The model under review builds one solid part; all positions refer to its coordinate system, in mm. A direction names the side the tool comes from. Coordinates: 2 decimals unless noted, no trailing zeros. Loops run counter-clockwise (first coordinate to the right, second up) from the corner with the lowest first, then second, coordinate; pieces in that order, holes last. Notation, with made-up numbers: M 34,16 L 45,16 A14 ccw 45,31 Z; hole C 20.25,79 d5. An arc over 180 degrees is marked long. One line per item, written item: value.
```python
from build123d import *

# Parameters (mm, degrees)
BOSS_EXTRUDE1_DEPTH = 33.6042
CUT_EXTRUDE1_DEPTH  = 1.397
CHAMFER1_SIZE       = 0.762
SKETCH3_W           = 18.6436
SKETCH3_H           = 2.4892
BOSS_EXTRUDE2_DEPTH = 6.604
SKETCH4_W           = 18.6436
SKETCH4_H           = 2.4892
BOSS_EXTRUDE3_DEPTH = 6.604
FILLET1_R           = 1.27
CUT_EXTRUDE2_DEPTH  = 3.048
SKETCH6_W           = 6.604
SKETCH6_H           = 1.2192
BOSS_EXTRUDE4_DEPTH = 1.905
CUT_EXTRUDE3_DEPTH  = 1.905
BOSS_EXTRUDE5_DEPTH = 3.0988
SKETCH9_R           = 6.731
BOSS_EXTRUDE6_DEPTH = 2.159
SKETCH10_R          = 4.9911
BOSS_EXTRUDE7_DEPTH = 0.508
SKETCH11_R          = 2.8702
BOSS_EXTRUDE8_DEPTH = 3.6576
SKETCH12_R          = 1.0668
CUT_EXTRUDE4_DEPTH  = 5.08
CHAMFER2_SIZE       = 0.254
SCALE1_SCALE        = 0.6


with BuildPart() as part:
    # Sketch1 → Boss-Extrude1 (new body)
    with BuildSketch(Plane(origin=(0, 0, 0), x_dir=(1, 0, 0), z_dir=(0, 1, 0))):
        with BuildLine():
            Line((0, 9.0424), (0, -9.0424))
            ThreePointArc((0, -9.0424), (0.29757951, -9.76082049), (1.016, -10.0584))
            Line((1.016, -10.0584), (39.116, -10.0584))
            ThreePointArc((39.116, -10.0584), (39.83442049, -9.76082049), (40.132, -9.0424))
            Line((40.132, -9.0424), (40.132, 9.0424))
            ThreePointArc((40.132, 9.0424), (39.83442049, 9.76082049), (39.116, 10.0584))
            Line((39.116, 10.0584), (1.016, 10.0584))
            ThreePointArc((1.016, 10.0584), (0.29757951, 9.76082049), (0, 9.0424))
        make_face()
    extrude(amount=BOSS_EXTRUDE1_DEPTH)

    # Sketch2 → Cut-Extrude1 (cut)
    with BuildSketch(Plane.XZ):
        with BuildLine():
            Line((4.6482, 10.0584), (4.6482, 7.3533))
            ThreePointArc((4.6482, 7.3533), (4.067919955, 5.952380045), (2.667, 5.3721))
            Line((2.667, 5.3721), (0, 5.3721))
            Line((0, 5.3721), (0, 9.0424))
            ThreePointArc((0, 9.0424), (0.29757951, 9.76082049), (1.016, 10.0584))
            Line((1.016, 10.0584), (4.6482, 10.0584))
        make_face()
        with BuildLine():
            Line((35.4838, 10.0584), (35.4838, 7.3533))
            ThreePointArc((35.4838, 7.3533), (36.064080045, 5.952380045), (37.465, 5.3721))
            Line((37.465, 5.3721), (40.132, 5.3721))
            Line((40.132, 5.3721), (40.132, 9.0424))
            ThreePointArc((40.132, 9.0424), (39.83442049, 9.76082049), (39.116, 10.0584))
            Line((39.116, 10.0584), (35.4838, 10.0584))
        make_face()
        with BuildLine():
            Line((0, -5.3721), (2.667, -5.3721))
            ThreePointArc((2.667, -5.3721), (4.067919955, -5.952380045), (4.6482, -7.3533))
            Line((4.6482, -7.3533), (4.6482, -10.0584))
            Line((4.6482, -10.0584), (1.016, -10.0584))
            ThreePointArc((1.016, -10.0584), (0.29757951, -9.76082049), (0, -9.0424))
            Line((0, -9.0424), (0, -5.3721))
        make_face()
        with BuildLine():
            Line((37.465, -5.3721), (40.132, -5.3721))
            Line((40.132, -5.3721), (40.132, -9.0424))
            ThreePointArc((40.132, -9.0424), (39.83442049, -9.76082049), (39.116, -10.0584))
            Line((39.116, -10.0584), (35.4838, -10.0584))
            Line((35.4838, -10.0584), (35.4838, -7.3533))
            ThreePointArc((35.4838, -7.3533), (36.064080045, -5.952380045), (37.465, -5.3721))
        make_face()
    extrude(amount=-CUT_EXTRUDE1_DEPTH, mode=Mode.SUBTRACT)

    # Chamfer1
    chamfer1_edges = [part.edges().sort_by_distance(p)[0] for p in [
        (20.066, 0, 10.0584),
        (0, 0, 0),
        (40.132, 0, 0),
        (20.066, 0, -10.0584),
    ]]
    chamfer(chamfer1_edges, length=CHAMFER1_SIZE)

    # Sketch3 → Boss-Extrude2 (add, symmetric)
    with BuildSketch(Plane(origin=(40.132, 0, 0), x_dir=(0, 0, -1), z_dir=(1, 0, 0))):
        with Locations((0, 27.4574)):
            Rectangle(SKETCH3_W, SKETCH3_H)
    extrude(amount=BOSS_EXTRUDE2_DEPTH, both=True)

    # Sketch4 → Boss-Extrude3 (add, symmetric)
    with BuildSketch(Plane.ZY):
        with Locations((0, 27.4574)):
            Rectangle(SKETCH4_W, SKETCH4_H)
    extrude(amount=BOSS_EXTRUDE3_DEPTH, both=True)

    # Fillet1
    fillet1_edges = [part.edges().sort_by_distance(p)[0] for p in [
        (46.736, 27.4574, 9.3218),
        (46.736, 27.4574, -9.3218),
        (-6.604, 27.4574, -9.3218),
        (-6.604, 27.4574, 9.3218),
    ]]
    fillet(fillet1_edges, radius=FILLET1_R)

    # Sketch5 → Cut-Extrude2 (cut)
    with BuildSketch(Plane(origin=(0, 28.702, 0), x_dir=(1, 0, 0), z_dir=(0, 1, 0))):
        with BuildLine():
            Line((-6.604, 3.4925), (-5.625185736, 3.4925))
            ThreePointArc((-5.625185736, 3.4925), (-1.7018, 4.9911), (-5.625185736, 6.4897))
            Line((-5.625185736, 6.4897), (-6.604, 6.4897))
            Line((-6.604, 6.4897), (-6.604, 3.4925))
        make_face()
        with BuildLine():
            Line((-6.604, -6.4897), (-5.625185736, -6.4897))
            ThreePointArc((-5.625185736, -6.4897), (-1.7018, -4.9911), (-5.625185736, -3.4925))
            Line((-5.625185736, -3.4925), (-6.604, -3.4925))
            Line((-6.604, -3.4925), (-6.604, -6.4897))
        make_face()
        with BuildLine():
            Line((45.757185736, -6.4897), (46.736, -6.4897))
            Line((46.736, -6.4897), (46.736, -3.4925))
            Line((46.736, -3.4925), (45.757185736, -3.4925))
            ThreePointArc((45.757185736, -3.4925), (41.8338, -4.9911), (45.757185736, -6.4897))
        make_face()
        with BuildLine():
            Line((45.757185736, 3.4925), (46.736, 3.4925))
            Line((46.736, 3.4925), (46.736, 6.4897))
            Line((46.736, 6.4897), (45.757185736, 6.4897))
            ThreePointArc((45.757185736, 6.4897), (41.8338, 4.9911), (45.757185736, 3.4925))
        make_face()
    extrude(amount=-CUT_EXTRUDE2_DEPTH, mode=Mode.SUBTRACT)

    # Sketch6 → Boss-Extrude4 (add)
    with BuildSketch(Plane(origin=(0, 28.702, 0), x_dir=(1, 0, 0), z_dir=(0, 1, 0))):
        with Locations((-3.302, 0)):
            Rectangle(SKETCH6_W, SKETCH6_H)
        with Locations((43.434, 0)):
            Rectangle(SKETCH6_W, SKETCH6_H)
    extrude(amount=BOSS_EXTRUDE4_DEPTH)

    # Sketch7 → Cut-Extrude3 (cut)
    with BuildSketch(Plane.XY.offset(0.6096)):
        Polygon((40.132, 30.607), (46.736, 28.702), (46.736, 30.607), align=None)
        Polygon((0, 30.607), (-6.604, 28.702), (-6.604, 30.607), align=None)
    extrude(amount=-CUT_EXTRUDE3_DEPTH, mode=Mode.SUBTRACT)

    # Sketch8 → Boss-Extrude5 (add)
    with BuildSketch(Plane(origin=(0, 33.6042, 0), x_dir=(1, 0, 0), z_dir=(0, 1, 0))):
        with BuildLine():
            Line((14.8583952, -8.8392), (34.1122, -8.8392))
            ThreePointArc((34.1122, -8.8392), (34.291805122, -8.764805122), (34.3662, -8.5852))
            Line((34.3662, -8.5852), (34.3662, -3.741254719))
            ThreePointArc((34.3662, -3.741254719), (36.053651663, 0), (34.3662, 3.741254719))
            Line((34.3662, 3.741254719), (34.3662, 8.5852))
            ThreePointArc((34.3662, 8.5852), (34.291805122, 8.764805122), (34.1122, 8.8392))
            Line((34.1122, 8.8392), (14.8583952, 8.8392))
            ThreePointArc((14.8583952, 8.8392), (0, 0), (14.8583952, -8.8392))
        make_face()
    extrude(amount=BOSS_EXTRUDE5_DEPTH)

    # Sketch9 → Boss-Extrude6 (add)
    with BuildSketch(Plane(origin=(0, 36.703, 0), x_dir=(1, 0, 0), z_dir=(0, 1, 0))):
        with Locations(Location((10.0584, 0, 0), (0, 0, 270))):
            Circle(SKETCH9_R)
    extrude(amount=BOSS_EXTRUDE6_DEPTH)

    # Sketch10 → Boss-Extrude7 (add)
    with BuildSketch(Plane(origin=(0, 38.862, 0), x_dir=(1, 0, 0), z_dir=(0, 1, 0))):
        with Locations(Location((10.0584, 0, 0), (0, 0, 270))):
            Circle(SKETCH10_R)
    extrude(amount=BOSS_EXTRUDE7_DEPTH)

    # Sketch11 → Boss-Extrude8 (add)
    with BuildSketch(Plane(origin=(0, 39.37, 0), x_dir=(1, 0, 0), z_dir=(0, 1, 0))):
        with Locations(Location((10.0584, 0, 0), (0, 0, 270))):
            Circle(SKETCH11_R)
    extrude(amount=BOSS_EXTRUDE8_DEPTH)

    # Sketch12 → Cut-Extrude4 (cut)
    with BuildSketch(Plane(origin=(0, 43.0276, 0), x_dir=(1, 0, 0), z_dir=(0, 1, 0))):
        with Locations(Location((10.0584, 0, 0), (0, 0, 270))):
            Circle(SKETCH12_R)
    extrude(amount=-CUT_EXTRUDE4_DEPTH, mode=Mode.SUBTRACT)

    # Chamfer2
    chamfer2_edges = [part.edges().sort_by_distance(p)[0] for p in [
        (10.0584, 43.0276, -2.8702),
        (10.0584, 43.0276, -1.0668),
    ]]
    chamfer(chamfer2_edges, length=CHAMFER2_SIZE)


with BuildPart() as part_1:
    # Scale1: scaled about (19.790017038, 18.508512474, 0)
    add(part.part.scale(SCALE1_SCALE).moved(Location((7.916006815, 7.40340499, 0))))


solid = part_1.part
```
(1) Draft analysis for pull direction X (two halves, no side actions). For faces 1 (the face through (20, 7.403, 0)), 2 (the face through (33.017, 23.888, 2.949)), 3 (the face through (35.958, 23.9, -4.4)), state which applies: pulls with the +X half, pulls with the -X half, needs draft (parallel to the pull), parting line crosses it, or undercut.
Checks:
face 1: needs draft
face 2: undercut
face 3: pulls with the +X half
(2) To check wall thickness, follow L1, parallel to X at y = 31.4, z = 0; L2, parallel to X at y = 26.75, z = 0.25; L3, parallel to Y at x = 20.5, z = -3.5. State the ranges of each line that lie inside material, in increasing order. Write a range as [from, to].
Checks:
L1: [12.23, 13.31], [14.59, 15.67]
L2: [7.92, 32]
L3: [7.4, 29.43]
(3) Add section C-C on x = 34. State the section outline as (y, z) points.
Checks:
outline: M 23.13,-5.59 L 24.62,-5.59 L 24.62,-4.29 L 23.13,-4.29 Z; M 23.13,-1.7 L 24.62,-1.7 L 24.62,-0.37 L 25.19,-0.37 L 25.19,0.37 L 24.62,0.37 L 24.62,1.7 L 23.13,1.7 Z; M 23.13,4.29 L 24.62,4.29 L 24.62,5.59 L 23.13,5.59 Z
(4) Add section A-A on y = 28.5. State the section outline as (x, z) points, then the cut area to 3 significant figures.
Checks:
outline: M 16.83,-5.3 L 28.38,-5.3 A0.15 ccw 28.54,-5.15 L 28.54,-2.24 A2.99 ccw 28.54,2.24 L 28.54,5.15 A0.15 ccw 28.38,5.3 L 16.83,5.3 A6.04 ccw long Z
area: 218 mm^2
(5) Tool access review of faces 4 (the face through (33, 24.625, 2)), 5 (the face through (10.366, 7.817, 3.581)), 6 (the face through (31, 8.242, 5)): name each direction out of +Z, -Z, +X, -X, +Y, -Y from which nothing blocks a thin tool from reaching the whole face with its end or side.
Checks:
face 4: +Z, +X, +Y
face 5: +Z, -X, -Y
face 6: +Z, +X, -Y
(6) Add section D-D on y = 12.25. State the section outline as (x, z) points, then the cut area to 3 significant figures.
Checks:
outline: M 7.92,-5.43 A0.61 ccw 8.53,-6.04 L 31.39,-6.04 A0.61 ccw 32,-5.43 L 32,5.43 A0.61 ccw 31.39,6.04 L 8.53,6.04 A0.61 ccw 7.92,5.43 Z
area: 290 mm^2
(7) Add section B-B on x = 20. State the section outline as (y, z) points.
Checks:
outline: M 7.4,-5.58 L 7.86,-6.04 L 27.57,-6.04 L 27.57,-5.3 L 29.43,-5.3 L 29.43,5.3 L 27.57,5.3 L 27.57,6.04 L 7.86,6.04 L 7.4,5.58 Z
(8) Insertion check: pin 1 Ø1.5 at (y, z) = (21.5, -0.5) entering from +X; pin 2 Ø2 at (x, z) = (6, 2) entering from +Y; pin 3 Ø0.7 at (y, z) = (7.5, 5) entering from +X. Each pin has a flat end and moves straight along its axis. Give the tip position at first contact, or say it passes through.
Checks:
pin 1: x = 32
pin 2: y = 24.62
pin 3: x = 29.21
